Geometry: see drawing. Coordinates: mm, zero at the bounding-box minimum. Round coordinates to 2 decimals unless told otherwise and drop trailing zeros. Loops run counter-clockwise (first coordinate to the right, second up) from the corner with the lowest first, then second, coordinate; pieces in that order, holes last.
(1) Cut plane C-C, the plane x = 70.5. Output: boundary loops of the cut face in (y, z), and give its area (3 significant figures).
(2) Cut plane A-A, the plane y = 6.25. Give the number of separate pieces and of enclosed holes in the cut face, and give its area (3 significant figures).
(3) First-contact query: pin 1 Ø3.5 at (x, z) = (350, 200) entering from -Y; pin 2 Ø10 at (x, y) = (524.5, 9.5) entering from +Z; pin 3 Ø5 at (x, y) = (299.5, 5) entering from +Z; pin 4 Ø1 at (x, y) = (334, 15) entering from +Z. Flat tips, straight axial feed; report the tip coordinate or a pass-through.
(4) Cut plane B-B, the plane z = 465. Output: boundary loops of the cut face in (x, y).
(5) Line query: line 1 (Z direction, x = 79.5, y = 11.5); line 2 (Z direction, x = 538.5, y = 12); line 3 (X direction, y = 12.75, z = 33). Output: solid intervals per line, ascending.
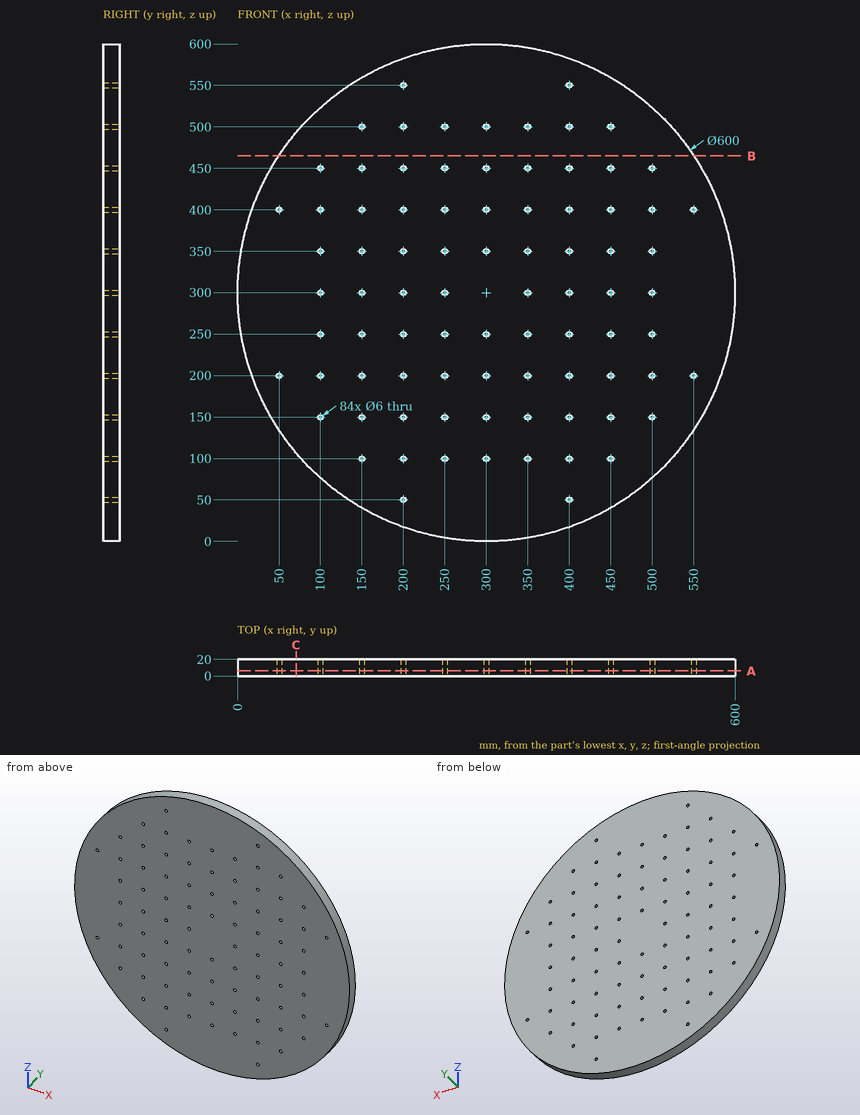
Reported:
1. outline: (0, 106.79) - (20, 106.79) - (20, 493.21) - (0, 493.21) - close
1. area: 7,730 mm2
2. separate pieces: 1
2. enclosed holes: 84
2. area: 280,000 mm2
3. pin 1: passes through
3. pin 2: stops at z = 504.5
3. pin 3: stops at z = 600
3. pin 4: stops at z = 598.12
4. outline: (49.45, 0) - (550.55, 0) - (550.55, 20) - (49.45, 20) - close
5. line 1: z = 96.58 to 503.42
5. line 2: z = 118.02 to 481.98
5. line 3: x = 163.21 to 436.79
